Autodesk Inventor part; units mm, degrees
ref_plane "YZ Plane" through (0, 0, 0) normal (1, 0, 0) x (0, 1, 0)
ref_plane "XZ Plane" through (0, 0, 0) normal (0, 1, 0) x (-1, 0, 0)
ref_plane "XY Plane" through (0, 0, 0) normal (0, 0, 1) x (1, 0, 0)
sketch "Sketch5" plane through (0, 0, 0) normal (0, 0, 1) x (1, 0, 0)
  line L0 (-30, 30) -> (30, 30)
  line L1 (30, 30) -> (30, -30)
  line L2 (30, -30) -> (-30, -30)
  line L3 (-30, -30) -> (-30, 30)
  point P0 (0, 0)
  point P1 (0, 30)
  point P2 (30, 0)
  dimension "d8" = 60
  dimension "d9" = 60
extrude "Extrusion5" add sketch "Sketch5" along normal blind 195
sketch "Sketch8" plane through (0, 0, 195) normal (0, 0, 1) x (1, 0, 0)
  line L0 (-30, -30) -> (30, -30)
  line L1 (30, -30) -> (30, 30)
  line L2 (-30, 30) -> (15, 30)
  line L3 (15, 30) -> (15, -15)
  line L4 (15, -15) -> (-30, -15)
  line L5 (-30, -15) -> (-30, 30)
  point P0 (0, 0)
  dimension "d25" = 15
  dimension "d26" = 15
extrude "Extrusion8" cut sketch "Sketch8" against normal blind 165
sketch "Sketch9" plane through (0, 0, 30) normal (0, 0, 1) x (1, 0, 0)
  circle A0 centre (6, 7.5) radius 4
  circle A1 centre (-21, 7.5) radius 4
  line L0 (30, -30) -> (30, 30)
  line L1 (-30, -30) -> (30, -30)
  circle A2 centre (6, 7.5) radius 8
  line L2 (-30, -15) -> (-30, 30)
  line L3 (15, 30) -> (15, -15)
  circle A3 centre (-7.5, -6) radius 4
  circle A4 centre (-7.5, 21) radius 4
  line L4 (15, -15) -> (-30, -15)
  point P0 (0, 0)
  point P1 (15, 7.5)
  point P2 (-30, 7.5)
  point P3 (-7.5, -15)
  dimension "d29" = 24
  dimension "d31" = 8
  dimension "d32" = 16
  dimension "d41" = 9
  dimension "d42" = 27
  dimension "d43" = 27
  dimension "d44" = 13.5
  dimension "d45" = 9
hole "Hole1" at (6, 7.5, 30) at (-21, 7.5, 30) at (-7.5, 21, 30) at (-7.5, -6, 30) direction (0, 0, -1) diameter 8.5 end through all
fillet "Fillet2" radius 4 1 edges at (-7.5, -15, 30)
sketch "Sketch10" plane through (15, -15, 195) normal (-1, 0, 0) x (0, 0, 1)
  line L0 (-165, 45) -> (0, 45)
  circle A0 centre (-27.5, 30) radius 4
  circle A1 centre (-27.5, 6) radius 4
  circle A2 centre (-82.5, 30) radius 4
  circle A3 centre (-82.5, 6) radius 4
  circle A4 centre (-137.5, 30) radius 4
  circle A5 centre (-137.5, 6) radius 4
  line L1 (-195, -15) -> (0, -15)
  line L2 (0, 45) -> (0, 0)
  line L3 (-165, 45) -> (-165, 4)
  point P0 (-195, 15)
  dimension "d47" = 15
  dimension "d48" = 21
  dimension "d49" = 8
  dimension "d57" = 27.5
  dimension "d58" = 55
  dimension "d59" = 55
  dimension "d60" = 27.5
hole "Hole2" at (15, 15, 167.5) at (15, -9, 167.5) at (15, 15, 112.5) at (15, -9, 112.5) at (15, -9, 57.5) at (15, 15, 57.5) direction (1, 0, 0) diameter 6.647 end through all
sketch "Sketch11" plane through (-30, -15, 195) normal (0, 1, 0) x (1, 0, 0)
  line L0 (45, 0) -> (0, 0)
  circle A0 centre (15, 137.5) radius 4
  circle A1 centre (39, 137.5) radius 4
  circle A2 centre (15, 82.5) radius 4
  circle A3 centre (39, 82.5) radius 4
  circle A4 centre (15, 27.5) radius 4
  circle A5 centre (39, 27.5) radius 4
  line L1 (60, 195) -> (60, 0)
  point P0 (30, 195)
  dimension "d63" = 8
  dimension "d65" = 55
  dimension "d66" = 55
  dimension "d68" = 24
  dimension "d69" = 21
  dimension "d70" = 27.5
hole "Hole3" at (9, -15, 167.5) at (-15, -15, 167.5) at (9, -15, 112.5) at (-15, -15, 112.5) at (9, -15, 57.5) at (-15, -15, 57.5) direction (0, -1, 0) diameter 6.647 end through all
sketch "Sketch12" plane through (-30, -30, 0) normal (-1, 0, 0) x (0, 0, 1)
  line L0 (195, 15) -> (195, 0)
  circle A0 centre (176.25, 7.5) radius 3
  circle A1 centre (106.25, 7.5) radius 3
  point P0 (0, 30)
  point P1 (195, 7.5)
  dimension "d78" = 70
  dimension "d79" = 18.75
  dimension "d80" = 6
hole "Hole4" at (-30, -22.5, 176.25) at (-30, -22.5, 106.25) direction (1, 0, 0) diameter 4.134 depth 15 tip angle 118
sketch "Sketch13" plane through (-30, 30, 0) normal (0, 1, 0) x (1, 0, 0)
  line L0 (60, -195) -> (45, -195)
  circle A0 centre (52.5, -176.25) radius 3
  circle A1 centre (52.5, -106.25) radius 3
  point P0 (30, 0)
  point P1 (52.5, -195)
  dimension "d88" = 18.75
  dimension "d89" = 70
  dimension "d90" = 6
hole "Hole5" at (22.5, 30, 176.25) at (22.5, 30, 106.25) direction (0, -1, 0) diameter 4.134 depth 15 tip angle 118
chamfer "Chamfer1" distance 5 angle 45 2 edges at (30, -30, 97.5) (-30, 30, 15)
chamfer "Chamfer2" distance 2 angle 45 2 edges at (30, 30, 97.5) (-30, -30, 97.5)
sketch "Sketch14" plane through (0, 0, 195) normal (0, 0, 1) x (1, 0, 0)
  line L0 (-28, -30) -> (25, -30)
  line L1 (30, -25) -> (30, 28)
  line L2 (15, -15) -> (-30, -15)
  circle A0 centre (15, -22.5) radius 2.5
  circle A1 centre (-23.5, -22.5) radius 2.5
  circle A2 centre (22.5, 23.5) radius 2.5
  line L3 (28, 30) -> (15, 30)
  line L4 (-30, -15) -> (-30, -28)
  circle A3 centre (22.5, -15) radius 2.5
  point P0 (0, 0)
  dimension "d104" = 15
  dimension "d105" = 7.5
  dimension "d106" = 5
  dimension "d107" = 7.5
  dimension "d116" = 6.5
  dimension "d117" = 6.5
  dimension "d119" = 45
  dimension "d120" = 45
hole "Hole6" at (-23.5, -22.5, 195) at (15, -22.5, 195) at (22.5, 23.5, 195) at (22.5, -15, 195) direction (0, 0, -1) diameter 4.134 depth 15 tip angle 118
equation "\"d26\" = d25"
equation "\"d44\" = 0.5 * d43"
equation "\"d107\" = d105"
equation "\"d117\" = d116"
equation "\"d120\" = d119"
properties part number "BC-10016" material "Alumínio 7075"
Part model, mm, in its own coordinate system. A direction names the side the tool comes from. Round coordinates to 2 decimals unless told otherwise and drop trailing zeros. Loops run counter-clockwise (first coordinate to the right, second up) from the corner with the lowest first, then second, coordinate; pieces in that order, holes last. Notation, with made-up numbers: (-29, 74) -> (17, 74) arc R21 cw to (17, 84) -> close; hole circle Ø6 at (59.5, -30.5). An arc over 180 degrees is marked (long way). Use a Markdown table: item, result.
1) Cut at C-C, the plane z = 99. List the corners of the cut face in (x, y), and give its area (3 significant figures).
The answers:
| item | result |
|---|---|
| outline | (-30, -28) -> (-28, -30) -> (25, -30) -> (30, -25) -> (30, 28) -> (28, 30) -> (15, 30) -> (15, -15) -> (-30, -15) -> close |
| area | 1,560 mm2 |
2) Probe line 1 (Y direction, x = 21, z = 112.5); line 2 (X direction, y = -24, z = 112.5); line 3 (Z direction, x = 12, y = -24.5). List the from-to ranges inside material, lowest first. Write a range as [from, to].
The answers:
| item | result |
|---|---|
| line 1 | y = [-30, -12.32], [-5.68, 11.68], [18.32, 30] |
| line 2 | x = [-30, -18.32], [-11.68, 5.68], [12.32, 30] |
| line 3 | z = [0, 56.07], [58.93, 111.07], [113.93, 166.07], [168.93, 195] |
3) Cut at A-A, the plane z = 57.5. List the corners of the cut face in (x, y), and give its area (3 significant figures).
The answers:
| item | result |
|---|---|
| outline | (-30, -28) -> (-28, -30) -> (-18.32, -30) -> (-18.32, -15) -> (-30, -15) -> close; (-11.68, -30) -> (5.68, -30) -> (5.68, -15) -> (-11.68, -15) -> close; (12.32, -30) -> (25, -30) -> (30, -25) -> (30, -12.32) -> (15, -12.32) -> (15, -15) -> (12.32, -15) -> close; (15, -5.68) -> (30, -5.68) -> (30, 11.68) -> (15, 11.68) -> close; (15, 18.32) -> (30, 18.32) -> (30, 28) -> (28, 30) -> (15, 30) -> close |
| area | 1,160 mm2 |
4) Drop flat-ended pins along their axis: pin 1 Ø10.5 at (y, z) = (15, 57.5) entering from -X; pin 2 Ø7.5 at (x, z) = (-15, 112.5) entering from +Y; pin 3 Ø3.5 at (y, z) = (-22.5, 106.25) entering from -X. Give the stop position or say it passes through.
The answers:
| item | result |
|---|---|
| pin 1 | stops at x = 15 |
| pin 2 | stops at y = -15 |
| pin 3 | stops at x = -14.81 |
5) Cut at B-B, the plane y = 7.5. List the corners of the cut face in (x, z), and give its area (4 significant figures).
The answers:
| item | result |
|---|---|
| outline | (-30, 0) -> (-25.25, 0) -> (-25.25, 30) -> (-30, 30) -> close; (-16.75, 0) -> (1.75, 0) -> (1.75, 30) -> (-16.75, 30) -> close; (10.25, 0) -> (30, 0) -> (30, 195) -> (15, 195) -> (15, 30) -> (10.25, 30) -> close |
| area | 3,765 mm2 |
6) Tool access for faces 1 (the cylindrical face through (21.88, 22.4, 178.22)), 2 (the cylindrical face through (14.38, -24.47, 187.4)), 3 (the cylindrical face through (-7.815, -13.797, 31.141)), 4 (the cylindrical face through (22.6, -10, 170.67)): list every direction of +Z, -Z, +X, -X, +Y, -Y with a clear straight run to the whole face (end or side of a thin tool).
The answers:
| item | result |
|---|---|
| face 1 | +Y |
| face 2 | +Z |
| face 3 | +Z, -X, +Y |
| face 4 | +X, -X |
7) Pull direction X, two halves, no side cores. Call faces 5 (the cylindrical face through (22.6, -6.98, 54.86)), 6 (the conical face through (15, -22.1, 179)), 7 (the flat face through (30, 2, 96)): pulls with the +X half, pulls with the -X half, needs draft (parallel to the pull), parting line crosses it, or undercut.
The answers:
| item | result |
|---|---|
| face 5 | needs draft |
| face 6 | undercut |
| face 7 | pulls with the +X half |
